Input: part model. Units: mm. Frame: model coordinates. A direction names the side the tool comes from. Give positions to 0.01 mm unless a question says otherwise; leave off trailing zeros. Write each loop counter-clockwise with the first axis right and the second up, starting at its lowest first coordinate (ties: lowest second). Pieces come first, ordered by that corner, then holes. Notation, with made-up numbers: M -4,76.25 L 0,76.25 A23 ccw 0,89.25 Z; hole C 4,-20 d10. An arc over 180 degrees is marked long. Use CSV: the item, a comma, the result in double quotes. Start each with the question number.
from build123d import *

# Parameters (mm, degrees)
FLANGE_BASE1_DEPTH = 2


# Sheet-metal steps are written as plain solids
with BuildPart() as part:
    # Esboço1 → Flange-base1 (new body)
    with BuildSketch(Plane(origin=(0, 0, 0), x_dir=(1, 0, 0), z_dir=(0, 1, 0))):
        Polygon((3, 37.500755799), (19, 37.500755799), (19, 27.500755799), (15, 25.500755799), (15, 19.500755799), (19, 17.500755799), (19, 0), (-19, 0), (-19, 17.500755799), (-15, 19.500755799), (-15, 25.500755799), (-19, 27.500755799), (-19, 37.500755799), (-3, 37.500755799), (-3, 27.500755799), (-7, 25.500755799), (-7, 19.500755799), (0, 16), (7, 19.500755799), (7, 25.500755799), (3, 27.500755799), align=None)
    extrude(amount=-FLANGE_BASE1_DEPTH)


solid = part.part
Q1. Section C-C, the plane y = -1.05. Return the cut outline in (x, z), and give its area (3 significant figures).
Q2. Material intervals for L1, parallel to X at y = -0.6, z = -30.5; L2, parallel to X at y = -0.25, z = -24; L3, parallel to Z at x = -16, y = -1.6, sorted ascending. Write a range as [from, to].
Q3. First-contact query: pin 1 Ø0.6 at (y, z) = (-1.5, -21.5) entering from +X; pin 2 Ø0.6 at (y, z) = (-1, -24) entering from -X. Flat tips, straight axial feed; report the tip coordinate or a pass-through.
Q4. Section A-A, the plane z = -28.5. Return the cut outline in (x, y), and give its area (3 significant figures).
Q5. Section B-B, the plane x = 4.5. Return the cut outline in (y, z).
Q6. Set-up query: faces 4 (the flat face through (-15, -1, -22)), 5 (the flat face through (3, -1, -32)), 6 (the flat face through (-5, -1, -26.5)). Return all of +Z, -Z, +X, -X, +Y, -Y with unobstructed straight access to the full face (end or side cutting, diameter ignored); none if empty.
Q7. Pull-direction query (X, two-part tool) for faces 1 (the flat face through (7, -1, -22)), 2 (the flat face through (19, -1, -9)), 3 (the flat face through (-17, -1, -18.5)); classes: released by +X, released by -X, zero draft, split by the parting line, or undercut.
Check result:
1,outline,"M -19,-37.5 L -3,-37.5 L -3,-27.5 L -7,-25.5 L -7,-19.5 L 0,-16 L 7,-19.5 L 7,-25.5 L 3,-27.5 L 3,-37.5 L 19,-37.5 L 19,-27.5 L 15,-25.5 L 15,-19.5 L 19,-17.5 L 19,0 L -19,0 L -19,-17.5 L -15,-19.5 L -15,-25.5 L -19,-27.5 Z"
1,area,"1,170 mm²"
2,L1,"x = [-19, -3], [3, 19]"
2,L2,"x = [-15, -7], [7, 15]"
2,L3,"z = [-37.5, -26], [-19, 0]"
3,pin 1,"stops at x = 15"
3,pin 2,"stops at x = -15"
4,outline,"M -19,-2 L -3,-2 L -3,0 L -19,0 Z; M 3,-2 L 19,-2 L 19,0 L 3,0 Z"
4,area,"64.0 mm²"
5,outline,"M -2,-37.5 L 0,-37.5 L 0,-26.75 L -2,-26.75 Z; M -2,-18.25 L 0,-18.25 L 0,0 L -2,0 Z"
6,face 4,"-X, +Y, -Y"
6,face 5,"-Z, +Y, -Y"
6,face 6,"+Y, -Y"
7,face 1,"undercut"
7,face 2,"released by +X"
7,face 3,"released by -X"
